from build123d import *

# Parameters (mm, degrees)
BASE_FLANGE1_DEPTH             = 170
EDGE_FLANGE1_STRIP_W           = 0.762
EDGE_FLANGE1_STRIP_H           = 0.127
EDGE_FLANGE1_STRIP_CUT_DEPTH   = 229.873
EDGE_FLANGE1_STRIP_2_W         = 0.762
EDGE_FLANGE1_STRIP_2_H         = 0.127
EDGE_FLANGE1_STRIP_CUT_2_DEPTH = 229.873
EDGE_FLANGE1_DEPTH             = 229.873
EDGE_FLANGE1_BEND_DEPTH        = 229.873
SKETCH19_W                     = 16.773112734
SKETCH19_H                     = 37.266497541
CUT_EXTRUDE1_DEPTH             = 10


# Sheet-metal steps are written as plain solids
with BuildPart() as part:
    # Sketch1 → Base-Flange1 (new body)
    with BuildSketch(Plane.XY):
        with BuildLine():
            Line((0, 0), (229.873, 0))
            ThreePointArc((229.873, 0), (229.962802561, 0.037197439), (230, 0.127))
            Line((230, 0.127), (230, 7))
            Line((230, 7), (230.127, 7))
            Line((230.127, 7), (230.127, 0.127))
            ThreePointArc((230.127, 0.127), (230.052605122, -0.052605122), (229.873, -0.127))
            Line((229.873, -0.127), (0, -0.127))
            Line((0, -0.127), (0, 0))
        make_face()
    extrude(amount=BASE_FLANGE1_DEPTH)

    # Edge-Flange1 strip (across the edge) → Edge-Flange1 strip cut (cut)
    with BuildSketch(Plane.ZY.offset(-229.873)):
        with Locations((-0.127, -0.0635)):
            Rectangle(EDGE_FLANGE1_STRIP_W, EDGE_FLANGE1_STRIP_H)
    extrude(amount=EDGE_FLANGE1_STRIP_CUT_DEPTH, mode=Mode.SUBTRACT)

    # Edge-Flange1 strip 2 (across the edge) → Edge-Flange1 strip cut 2 (cut)
    with BuildSketch(Plane(origin=(0, 0, 170), x_dir=(0, 0, -1), z_dir=(1, 0, 0))):
        with Locations((-0.127, -0.0635)):
            Rectangle(EDGE_FLANGE1_STRIP_2_W, EDGE_FLANGE1_STRIP_2_H)
    extrude(amount=EDGE_FLANGE1_STRIP_CUT_2_DEPTH, mode=Mode.SUBTRACT)

    # Edge-Flange1 section (across the edge) → Edge-Flange1 (add)
    with BuildSketch(Plane.ZY.offset(-229.873)):
        with BuildLine():
            Line((0, 0.127), (0, 6.873))
            Line((0, 6.873), (0.127, 6.873))
            Line((0.127, 6.873), (0.127, 0.127))
            ThreePointArc((0.127, 0.127), (0.164197439, 0.037197439), (0.254, 0))
            Line((0.254, 0), (0.254, -0.127))
            ThreePointArc((0.254, -0.127), (0.074394878, -0.052605122), (0, 0.127))
        make_face()
    extrude(amount=EDGE_FLANGE1_DEPTH)

    # Edge-Flange1 section 2 (across the edge) → Edge-Flange1 bend (add)
    with BuildSketch(Plane(origin=(0, 0, 170), x_dir=(0, 0, -1), z_dir=(1, 0, 0))):
        with BuildLine():
            Line((0, 0.127), (0, 6.873))
            Line((0, 6.873), (0.127, 6.873))
            Line((0.127, 6.873), (0.127, 0.127))
            ThreePointArc((0.127, 0.127), (0.164197439, 0.037197439), (0.254, 0))
            Line((0.254, 0), (0.254, -0.127))
            ThreePointArc((0.254, -0.127), (0.074394878, -0.052605122), (0, 0.127))
        make_face()
    extrude(amount=EDGE_FLANGE1_BEND_DEPTH)

    # Sketch19 → Cut-Extrude1 (cut)
    with BuildSketch(Plane(origin=(0, 0, 0), x_dir=(1, 0, 0), z_dir=(0, 1, 0))):
        with Locations((8.386556367, -31.778783199)):
            Rectangle(SKETCH19_W, SKETCH19_H)
    extrude(amount=-CUT_EXTRUDE1_DEPTH, mode=Mode.SUBTRACT)


solid = part.part
Could you check a few things on this model? Use its own coordinates, in mm. Coordinates: 2 decimals unless noted, no trailing zeros. Loops run counter-clockwise (first coordinate to the right, second up) from the corner with the lowest first, then second, coordinate; pieces in that order, holes last.
1. For P1, Ø2, axis at x = 79.5, z = 85, coming from the +Y side; P2, Ø4, axis at y = 4, z = 54, coming from the -X side, each with a flat end and sliding along its axis, tell me the tip position at first contact or that it passes through.
2. Imagine slicing it at C-C (x = 205.5). Please give me the cut outline in (y, z), and give its area (3 significant figures).
3. Imagine slicing it at D-D (z = 104). Please give me the cut outline in (x, y), and give its area (3 significant figures).
4. Imagine slicing it at B-B (z = 42). Please give me the cut outline in (x, y).
5. Imagine slicing it at A-A (y = 5.5). Please give me the cut outline in (x, z).
Computed values:
1. P1: stops at y = 0
1. P2: stops at x = 230
2. outline: (-0.13, 0.25) arc R0.25 ccw to (0.13, 0) - (6.87, 0) - (6.87, 0.13) - (0.13, 0.13) arc R0.13 cw to (0, 0.25) - (0, 169.75) arc R0.13 cw to (0.13, 169.87) - (6.87, 169.87) - (6.87, 170) - (0.13, 170) arc R0.25 ccw to (-0.13, 169.75) - close
2. area: 23.3 mm2
3. outline: (0, -0.13) - (229.87, -0.13) arc R0.25 ccw to (230.13, 0.13) - (230.13, 7) - (230, 7) - (230, 0.13) arc R0.13 cw to (229.87, 0) - (0, 0) - close
3. area: 30.1 mm2
4. outline: (16.77, -0.13) - (229.87, -0.13) arc R0.25 ccw to (230.13, 0.13) - (230.13, 7) - (230, 7) - (230, 0.13) arc R0.13 cw to (229.87, 0) - (16.77, 0) - close
5. outline: (0, 0) - (229.87, 0) - (229.87, 0.13) - (0, 0.13) - close; (0, 169.87) - (229.87, 169.87) - (229.87, 170) - (0, 170) - close; (230, 0) - (230.13, 0) - (230.13, 170) - (230, 170) - close
